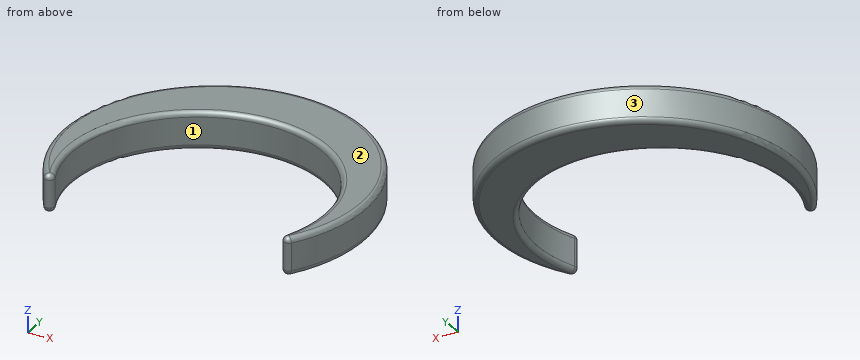
```python
from build123d import *

# Parameters (mm, degrees)
SKETCH_R     = 12
PAD_DEPTH    = 3
SKETCH001_R  = 10
POCKET_DEPTH = 3.001
FILLET_R     = 0.4


with BuildPart() as part:
    # Sketch → Pad (new body)
    with BuildSketch(Plane.XY):
        Circle(SKETCH_R)
    extrude(amount=PAD_DEPTH)

    # Sketch001 → Pocket (cut, through all)
    with BuildSketch(Plane.XY):
        with Locations((0, -2.467762)):
            Circle(SKETCH001_R)
    extrude(amount=POCKET_DEPTH, mode=Mode.SUBTRACT)

    # Fillet
    fillet_edges = [part.edges().sort_by_distance(p)[0] for p in [
        (-5.794891, 10.508056, 3),
        (-4.240751, 6.588508, 3),
        (-5.794891, 10.508056, 0),
        (-4.240751, 6.588508, 0),
        (9.05627, -6.708513, 0),
        (10.508056, -5.794891, 0),
        (6.403207, -10.14884, 1.5),
        (-6.403207, -10.14884, 1.5),
    ]]
    fillet(fillet_edges, radius=FILLET_R)


solid = part.part
```
Model file for the job. Use its own axes, mm. Face numbers are marked on the shaded views. Give positions to 0.01 mm unless a question says otherwise; leave off trailing zeros. Write each loop counter-clockwise with the first axis right and the second up, starting at its lowest first coordinate (ties: lowest second). Pieces come first, ordered by that corner, then holes. Notation, with made-up numbers: (56.5, 88) - (72.5, 88) arc R23 cw to (72.5, 98) - close; hole circle Ø6 at (4, 0.25). An arc over 180 degrees is marked (long way). One line per question, with ' | ' between items. Start each with the question number.
(1) Slice it at A-A on x = 0. Write the cut outline in (y, z).
(2) Two-plate mould, pull along Y, no slides. Class the marked faces 1, 2 and 3: +Y half, -Y half, draft (parallel to the pull), parting line (faces both ways), or undercut.
(3) Wall check: line 1 along X through (y, z) = (5, 0.7); line 2 along Y through (x, z) = (-0.25, 0.4); line 3 along X through (y, z) = (3, 0.45). Give the ranges that are in metal, low to high. Write a range as from..to.
Results below:
1) outline: (7.53, 0.4) arc R0.4 ccw to (7.93, 0) - (11.6, 0) arc R0.4 ccw to (12, 0.4) - (12, 2.6) arc R0.4 ccw to (11.6, 3) - (7.93, 3) arc R0.4 ccw to (7.53, 2.6) - close
2) face 1: undercut | face 2: draft | face 3: parting line
3) line 1: -10.91..-6.65, 6.65..10.91 | line 2: 7.53..12 | line 3: -11.62..-8.37, 8.37..11.62
